Could you check a few things on this drawing? It's one solid part, dimensions in mm from its lowest x, y, z. Coordinates: 2 decimals unless noted, no trailing zeros. Loops run counter-clockwise (first coordinate to the right, second up) from the corner with the lowest first, then second, coordinate; pieces in that order, holes last.
1) Imagine slicing it at D-D on x = 70. Please give me the cut outline in (y, z).
2) Imagine slicing it at C-C on z = 53.5. Please give me the cut outline in (x, y).
3) Imagine slicing it at A-A on x = 28. Please give me the cut outline in (y, z), plus the area to 3 significant figures.
4) Imagine slicing it at B-B on y = 22. Give the number of separate pieces and of enclosed holes in the cut face, plus the area to 3 significant figures.
5) If I drill on line 1 along Z through (x, y) = (51, 10.75); line 2 along X through (y, z) = (24, 60.5); line 3 along X through (y, z) = (7, 53.5), over which ranges is the centre line in solid material (lowest first)?
6) Will these pins go through, and if not, where does the flat tip stop? P1, Ø12, axis at y = 15, z = 26, coming from the -X side; P2, Ø6, axis at x = 99.5, z = 23.5, coming from the -Y side; P3, Ø1, axis at y = 19, z = 38.5, coming from the +X side; P4, Ø8, axis at y = 13, z = 81, coming from the -X side.
7) Thinking about a two-plate mould opening in Z: for the marked faces 1, 2, 3 and 4, which applies, released by +Z, released by -Z, zero draft, split by the parting line, or undercut?
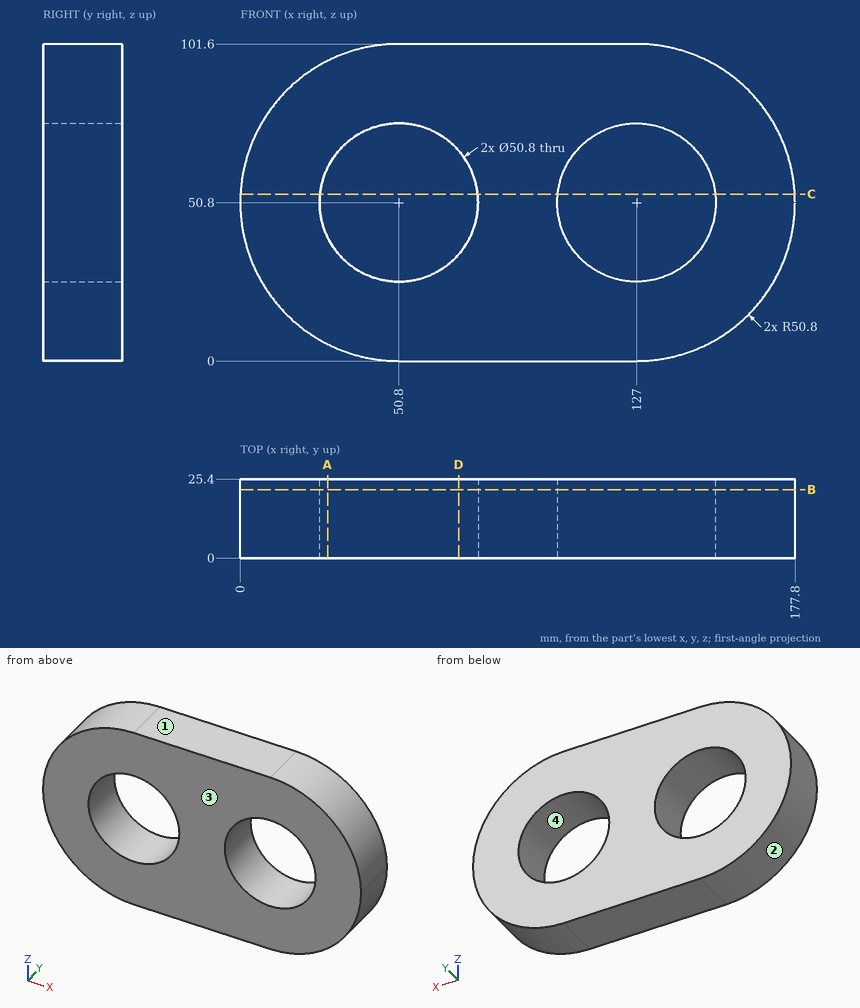
Filled in:
1. outline: (0, 0) - (25.4, 0) - (25.4, 34.17) - (0, 34.17) - close; (0, 67.43) - (25.4, 67.43) - (25.4, 101.6) - (0, 101.6) - close
2. outline: (0.07, 0) - (25.54, 0) - (25.54, 25.4) - (0.07, 25.4) - close; (76.06, 0) - (101.74, 0) - (101.74, 25.4) - (76.06, 25.4) - close; (152.26, 0) - (177.73, 0) - (177.73, 25.4) - (152.26, 25.4) - close
3. outline: (0, 5.4) - (25.4, 5.4) - (25.4, 39.61) - (0, 39.61) - close; (0, 61.99) - (25.4, 61.99) - (25.4, 96.2) - (0, 96.2) - close
3. area: 1,740 mm2
4. separate pieces: 1
4. enclosed holes: 2
4. area: 11,800 mm2
5. line 1: z = 0 to 25.4, 76.2 to 101.6
5. line 2: x = 0.93 to 27.33, 74.27 to 103.53, 150.47 to 176.87
5. line 3: x = 0.07 to 25.54, 76.06 to 101.74, 152.26 to 177.73
6. P1: stops at x = 3.61
6. P2: stops at y = 0
6. P3: stops at x = 176.41
6. P4: stops at x = 7.28
7. face 1: released by +Z
7. face 2: split by the parting line
7. face 3: zero draft
7. face 4: undercut
